Work out the finished part from the listing and answer in its coordinate system (mm). A direction names the side the tool comes from. Round coordinates to 2 decimals unless told otherwise and drop trailing zeros. Order: outer loops, then holes, each group sorted by start corner. A loop starts at its lowest first (then second) coordinate and runs counter-clockwise, first axis right, second up. Notation, with made-up numbers: M 15,10 L 61,10 A29 cw 61,48 Z; hole C 29.25,22.5 d9. An arc over 180 degrees is marked long. Answer as a JSON object with one key per item and string values. Group by question number.
from build123d import *

# Parameters (mm, degrees)
PAD_DEPTH        = 10
SKETCH001_R      = 3.05
POCKET_DEPTH     = 10.001
FILLET_R         = 2
FILLET001_R      = 2
HOLE_D           = 6.6
HOLE_DEPTH       = 25
HOLE_CBORE_D     = 11
HOLE_CBORE_DEPTH = 6.4


with BuildPart() as part:
    # Sketch → Pad (new body)
    with BuildSketch(Plane.XY):
        with BuildLine():
            Line((-45.5, 24), (45.5, 24))
            ThreePointArc((48.5, 21), (47.62132, 23.12132), (45.5, 24))
            Line((48.5, 21), (48.5, -21))
            ThreePointArc((45.5, -24), (47.62132, -23.12132), (48.5, -21))
            Line((45.5, -24), (-45.5, -24))
            ThreePointArc((-48.5, -21), (-47.62132, -23.12132), (-45.5, -24))
            Line((-48.5, -21), (-48.5, 21))
            ThreePointArc((-45.5, 24), (-47.62132, 23.12132), (-48.5, 21))
        make_face()
        with BuildLine():
            ThreePointArc((40.55, 13), (37.5, 16.05), (34.45, 13))
            Line((34.45, 13), (34.45, -13))
            ThreePointArc((34.45, -13), (37.5, -16.05), (40.55, -13))
            Line((40.55, -13), (40.55, 13))
        make_face(mode=Mode.SUBTRACT)
        with BuildLine():
            ThreePointArc((-34.45, 13), (-37.5, 16.05), (-40.55, 13))
            Line((-40.55, 13), (-40.55, -13))
            ThreePointArc((-40.55, -13), (-37.5, -16.05), (-34.45, -13))
            Line((-34.45, -13), (-34.45, 13))
        make_face(mode=Mode.SUBTRACT)
    extrude(amount=PAD_DEPTH)

    # Sketch001 (on Face18 of Pad) → Pocket (cut, through all)
    with BuildSketch(Plane.XY.offset(10)):
        with Locations((-12.5, 12.5)):
            Circle(SKETCH001_R)
        with Locations((12.5, 12.5)):
            Circle(SKETCH001_R)
        with Locations((-12.5, -12.5)):
            Circle(SKETCH001_R)
        with Locations((12.5, -12.5)):
            Circle(SKETCH001_R)
    extrude(amount=-POCKET_DEPTH, mode=Mode.SUBTRACT)

    # Fillet
    fillet_edges = [part.edges().sort_by_distance(p)[0] for p in [
        (0, -24, 10),
    ]]
    fillet(fillet_edges, radius=FILLET_R)

    # Fillet001
    fillet001_edges = [part.edges().sort_by_distance(p)[0] for p in [
        (0, -24, 0),
    ]]
    fillet(fillet001_edges, radius=FILLET001_R)

    # Hole
    with Locations(Plane.XY.offset(10)):
        with Locations((0, 0)):
            CounterBoreHole(HOLE_D / 2, HOLE_CBORE_D / 2, HOLE_CBORE_DEPTH, depth=HOLE_DEPTH)


solid = part.part
Item 1: Find section D-D (x = -12.5). Give the vertices of the cut face in (y, z).
Item 2: A tool of negligible diameter and unlimited length cuts with its end or side. For faces 1 (the cylindrical face through (47.64, 23.1, 4.96)), 2 (the flat face through (40.55, 0, 5)), from which of +Z, -Z, +X, -X, +Y, -Y can it reach the whole face along a straight path? Write none if from no direction.
Item 3: Find section A-A (z = 5.75). Give the vertices of the cut face in (x, y), and give its area (3 significant figures).
Item 4: Find section B-B (x = 37.5). Give the vertices of the cut face in (y, z), and give its area (3 significant figures).
Item 5: Find section C-C (y = -14.5). Give the vertices of the cut face in (x, z), and give its area (3 significant figures).
Item 6: Consider L1, parallel to Y at x = 12.5, z = 4; L2, parallel to X at y = 13.5, z = 3.5; L3, parallel to Y at x = 37.5, z = 2.25. Determine where each line is inside the solid, lowest interval first.
Item 7: The mould has two halves that part along Y. Classify faces 3 (the cylindrical face through (-0.64, -23.4, 9.43)), 4 (the cylindrical face through (0.64, 23.4, 9.43)), 5 (the cylindrical face through (-37.43, 16.05, 4.93)), 6 (the flat face through (1, -9, 10)): +Y half, -Y half, draft (parallel to the pull), parting line (faces both ways), or undercut.
Item 8: This flat-tipped pin is pushed along its axis until it touches: pin 1 (5.5 mm diameter, centred on x = 2.5, y = 0, fed in from +Z). Where does it stop, or does it pass through?
Responses:
{
 "1": {"outline": "M -24,2 A2 ccw -22,0 L -15.55,0 L -15.55,10 L -22,10 A2 ccw -24,8 Z; M -9.45,0 L 9.45,0 L 9.45,10 L -9.45,10 Z; M 15.55,0 L 22,0 A2 ccw 24,2 L 24,8 A2 ccw 22,10 L 15.55,10 Z"},
 "2": {"face 1": "+Z, -Z, +X, +Y", "face 2": "+Z, -Z"},
 "3": {"outline": "M -48.5,-21 A3 ccw -45.5,-24 L 45.5,-24 A3 ccw 48.5,-21 L 48.5,21 A3 ccw 45.5,24 L -45.5,24 A3 ccw -48.5,21 Z; hole M -40.55,-13 A3.05 ccw -34.45,-13 L -34.45,13 A3.05 ccw -40.55,13 Z; hole C -12.5,-12.5 d6.1; hole C -12.5,12.5 d6.1; hole C 0,0 d11; hole C 12.5,-12.5 d6.1; hole C 12.5,12.5 d6.1; hole M 34.45,-13 A3.05 ccw 40.55,-13 L 40.55,13 A3.05 ccw 34.45,13 Z", "area": "4,060 mm^2"},
 "4": {"outline": "M -24,2 A2 ccw -22,0 L -16.05,0 L -16.05,10 L -22,10 A2 ccw -24,8 Z; M 16.05,0 L 22,0 A2 ccw 24,2 L 24,8 A2 ccw 22,10 L 16.05,10 Z", "area": "156 mm^2"},
 "5": {"outline": "M -48.5,2 A2 ccw -46.5,0 L -40.16,0 L -40.16,10 L -46.5,10 A2 ccw -48.5,8 Z; M -34.84,0 L -14.8,0 L -14.8,10 L -34.84,10 Z; M -10.2,0 L 10.2,0 L 10.2,10 L -10.2,10 Z; M 14.8,0 L 34.84,0 L 34.84,10 L 14.8,10 Z; M 40.16,0 L 46.5,0 A2 ccw 48.5,2 L 48.5,8 A2 ccw 46.5,10 L 40.16,10 Z", "area": "768 mm^2"},
 "6": {"L1": "y = -24 to -15.55, -9.45 to 9.45, 15.55 to 24", "L2": "x = -48.5 to -40.51, -34.49 to -15.38, -9.62 to 9.62, 15.38 to 34.49, 40.51 to 48.5", "L3": "y = -24 to -16.05, 16.05 to 24"},
 "7": {"face 3": "-Y half", "face 4": "+Y half", "face 5": "undercut", "face 6": "draft"},
 "8": {"pin 1": "stops at z = 3.6"}
}
